The figure shows three views and two pictorial views of one solid part (mm, origin at its lowest corner). Answer the questions. A direction names the side the tool comes from. Coordinates: 2 decimals unless noted, no trailing zeros. Order: outer loops, then holes, each group sorted by start corner. A loop starts at its lowest first (then second) coordinate and runs counter-clockwise, first axis right, second up. Notation, with made-up numbers: (60.5, -22) - (90.5, -22) arc R16 ccw to (90.5, 3) - close; hole circle Ø2 at (-31, 44). An arc over 180 degrees is marked (long way). Answer as a JSON object with one key per item and string values. Group by question number.
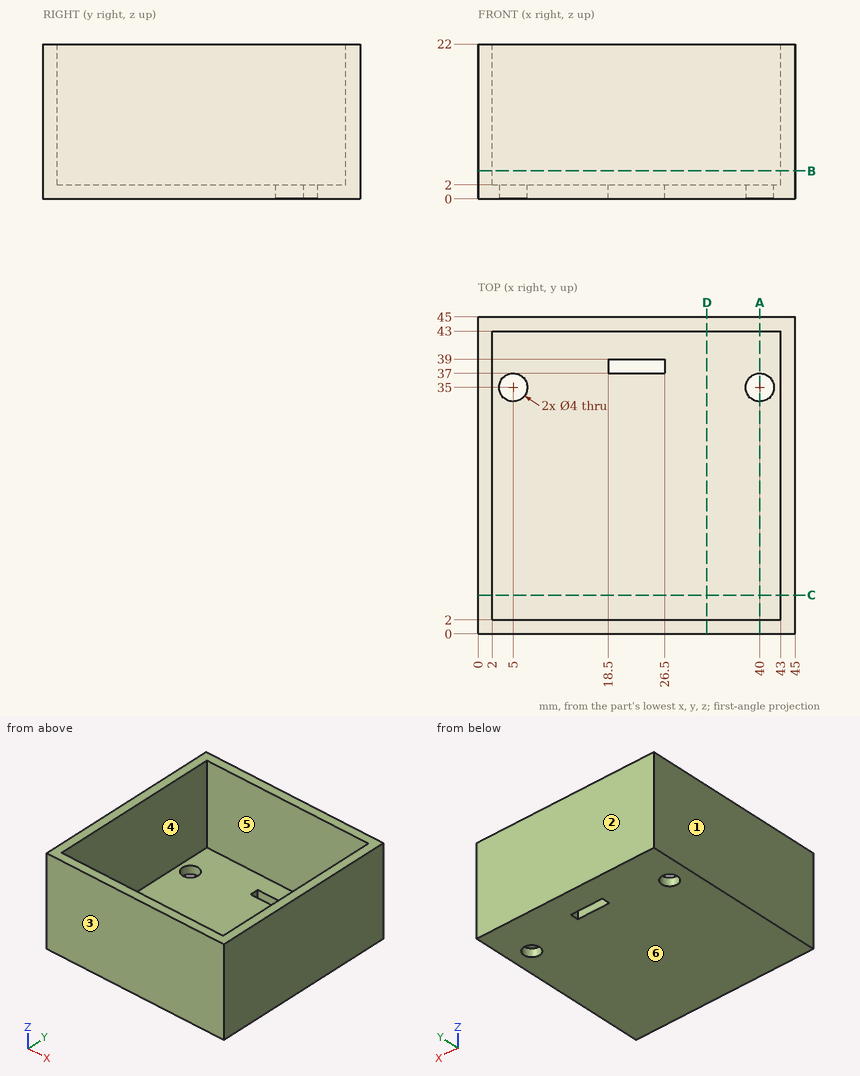
1. A cutting plane is placed at C-C on y = 5.5. Write down the section's boundary in (x, z).
2. Straight lines are drawn through the part: L1, parallel to X at y = 35, z = 1.1; L2, parallel to X at y = 35, z = 2.5; L3, parallel to Y at x = 40, z = 1.4. For each, find the intervals that lie inside material, in ascending order.
3. For the marked faces 5 and 6, determine the directions among +Z, -Z, +X, -X, +Y, -Y from which every point of the face is accessible in a straight line to the end or side of a thin tool.
4. For a pull along Y with two mould halves and no side action, classify the marked faces 1, 2, 3 and 4 as pulls with the +Y half, pulls with the -Y half, needs draft (parallel to the pull), parting line crosses it, or undercut.
5. A cutting plane is placed at A-A on x = 40. Write down the section's boundary in (y, z).
6. A cutting plane is placed at B-B on z = 4. Write down the section's boundary in (x, y).
Derived:
{
 "1": {"outline": "(0, 0) - (45, 0) - (45, 22) - (43, 22) - (43, 2) - (2, 2) - (2, 22) - (0, 22) - close"},
 "2": {"L1": "x = 0 to 3, 7 to 38, 42 to 45", "L2": "x = 0 to 2, 43 to 45", "L3": "y = 0 to 33, 37 to 45"},
 "3": {"face 5": "+Z", "face 6": "-Z, +X, -X, +Y, -Y"},
 "4": {"face 1": "needs draft", "face 2": "pulls with the +Y half", "face 3": "pulls with the -Y half", "face 4": "undercut"},
 "5": {"outline": "(0, 0) - (33, 0) - (33, 2) - (2, 2) - (2, 22) - (0, 22) - close; (37, 0) - (45, 0) - (45, 22) - (43, 22) - (43, 2) - (37, 2) - close"},
 "6": {"outline": "(0, 0) - (45, 0) - (45, 45) - (0, 45) - close; hole (2, 2) - (43, 2) - (43, 43) - (2, 43) - close"}
}
